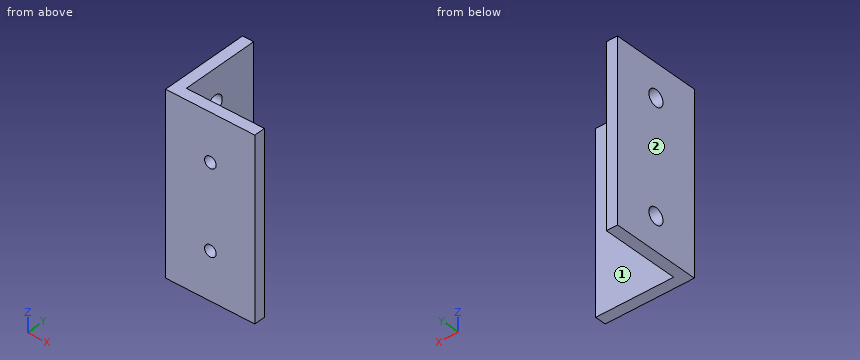
from build123d import *

# Parameters (mm, degrees)
BOSS_EXTRUDE1_DEPTH = 50.8
SKETCH2_R           = 1.65
CUT_EXTRUDE1_DEPTH  = 61.989758362
SKETCH3_R           = 2.3241
CUT_EXTRUDE2_DEPTH  = 63.217039467


with BuildPart() as part:
    # Sketch1 → Boss-Extrude1 (new body)
    with BuildSketch(Plane.XY):
        Polygon((0, 25.4), (0, 0), (25.4, 0), (25.4, 3.175), (3.175, 3.175), (3.175, 25.4), align=None)
    extrude(amount=BOSS_EXTRUDE1_DEPTH)

    # Sketch2 → Cut-Extrude1 (cut, through all)
    with BuildSketch(Plane(origin=(0, 3.175, 0), x_dir=(1, 0, 0), z_dir=(0, 1, 0))):
        with Locations(Location((12.75, -13.499999988, 0), (0, 0, 270))):
            Circle(SKETCH2_R)
        with Locations(Location((12.75, -37.299999988, 0), (0, 0, 270))):
            Circle(SKETCH2_R)
    extrude(amount=-CUT_EXTRUDE1_DEPTH, mode=Mode.SUBTRACT)

    # Sketch3 → Cut-Extrude2 (cut, through all)
    with BuildSketch(Plane.ZY):
        with Locations((9.525, 12.7)):
            Circle(SKETCH3_R)
        with Locations((41.275, 12.7)):
            Circle(SKETCH3_R)
    extrude(amount=-CUT_EXTRUDE2_DEPTH, mode=Mode.SUBTRACT)


solid = part.part
Work out the finished part from the listing and answer in its coordinate system (mm). Face numbers are marked on the shaded views. A direction names the side the tool comes from. Coordinates: 2 decimals unless noted, no trailing zeros. Write each loop counter-clockwise with the first axis right and the second up, starting at its lowest first coordinate (ties: lowest second). Pieces come first, ordered by that corner, then holes. Notation, with made-up numbers: M 31.25,8 L 55.25,8 A13 ccw 55.25,16 Z; hole C 59,-6 d3. An arc over 180 degrees is marked long. Answer as CSV lines item,"result". Start each with the question number.
Item 1: A tool of negligible diameter and unlimited length cuts with its end or side. For the marked faces 1 and 2, from which of +Z, -Z, +X, -X, +Y, -Y can it reach the whole face along a straight path? Write none if from no direction.
Item 2: Consider L1, parallel to X at y = 0.95, z = 37.3; L2, parallel to X at y = 21.25, z = 3 (3 decimals). Determine where each line is inside the solid, lowest interval first.
Item 3: Section B-B on y = 12.7 is taken. Write down the section's boundary in (x, z) (3 decimals), and give its area (3 significant figures).
Item 4: Section A-A on z = 13.5 is taken. Write down the section's boundary in (x, y) (3 decimals).
Item 5: Section D-D on x = 2.5 is taken. Write down the section's boundary in (y, z) (3 decimals), and give its area (3 significant figures).
Item 6: Flat-ended cylindrical pins translate along their axes: P1, Ø3.5, axis at y = 12.7, z = 9.525, coming from the -X side; P2, Ø5, axis at y = 13, z = 6, coming from the +X side (3 decimals); P3, Ø5, axis at x = 4, y = 8.5, coming from the +Z side; P4, Ø1, axis at x = 18.5, z = 11.5, coming from the +Y side (3 decimals). Find the tip coordinate at first contact, or state that the pin passes through.
Item 7: Section C-C on x = 12.75 is taken. Write down the section's boundary in (y, z) (3 decimals).
Checks:
1,face 1,"+Z, -Z, +X, +Y"
1,face 2,"+Z, -Z, -X, +Y, -Y"
2,L1,"x = 0 to 11.1, 14.4 to 25.4"
2,L2,"x = 0 to 3.175"
3,outline,"M 0,0 L 3.175,0 L 3.175,7.201 L 0,7.201 Z; M 0,11.849 L 3.175,11.849 L 3.175,38.951 L 0,38.951 Z; M 0,43.599 L 3.175,43.599 L 3.175,50.8 L 0,50.8 Z"
3,area,"132 mm²"
4,outline,"M 0,0 L 11.1,0 L 11.1,3.175 L 3.175,3.175 L 3.175,25.4 L 0,25.4 Z; M 14.4,0 L 25.4,0 L 25.4,3.175 L 14.4,3.175 Z"
5,outline,"M 0,0 L 25.4,0 L 25.4,50.8 L 0,50.8 Z; hole C 12.7,9.525 d4.648; hole C 12.7,41.275 d4.648"
5,area,"1,260 mm²"
6,P1,"passes through"
6,P2,"stops at x = 3.175"
6,P3,"stops at z = 50.8"
6,P4,"stops at y = 3.175"
7,outline,"M 0,0 L 3.175,0 L 3.175,11.85 L 0,11.85 Z; M 0,15.15 L 3.175,15.15 L 3.175,35.65 L 0,35.65 Z; M 0,38.95 L 3.175,38.95 L 3.175,50.8 L 0,50.8 Z"
